The listing builds one solid part. Answer for the finished solid, in the listing's coordinates (mm). A direction names the side the tool comes from. Round coordinates to 2 decimals unless told otherwise and drop trailing zeros. Write each loop counter-clockwise with the first axis right and the second up, starting at its lowest first coordinate (ties: lowest second). Pieces come first, ordered by that corner, then holes. Notation, with made-up numbers: (-1.75, -21.75) - (4.25, -21.75) arc R22 ccw to (4.25, 9.25) - close; hole circle Ø11 at (76.25, -21). An arc over 180 degrees is marked (long way). Answer as CSV lines item,"result". Start each with the question number.
Item 1: A cutting plane is placed at A-A on y = 20. Determine the outline of the cut face in (x, z), and give its area (3 significant figures).
Item 2: For a pull along Y with two mould halves and no side action, classify faces 1 (the flat face through (37.5, -1, 33)), 2 (the cylindrical face through (70.5, 71, 1.5)), 3 (the flat face through (-34.5, 0, 32)), 4 (the flat face through (-1, 37.5, 33)) as pulls with the +Y half, pulls with the -Y half, needs draft (parallel to the pull), parting line crosses it, or undercut.
Item 3: Straight lines are drawn through the part: line 1 along Y through (x, z) = (72, 1); line 2 along Y through (x, z) = (72.5, 2). For each, find the intervals that lie inside material, in ascending order. Write a range as [from, to].
Item 4: A cutting plane is placed at B-B on x = -72.5. Determine the outline of the cut face in (y, z), and give its area (3 significant figures).
Item 5: A cutting plane is placed at C-C on z = 21. Determine the outline of the cut face in (x, y).
Item 6: Flat-ended cylindrical pins translate along their axes: pin 1 (4 mm diameter, centred on y = -4, z = 16, fed in from -X); pin 2 (4 mm diameter, centred on x = -29.5, z = 31.5, fed in from +Y); pin 3 (18 mm diameter, centred on x = -18.5, z = 42.5, fed in from -Y); pin 4 (6 mm diameter, centred on x = -72.5, y = -72.5, fed in from -Z). Find the tip coordinate at first contact, or state that the pin passes through.
Item 7: Which of the six approach directions +Z, -Z, +X, -X, +Y, -Y give full straight-line access (tool end or side, diameter ignored) to faces 5 (the flat face through (34.5, 0, 32)), 6 (the flat face through (-3, -36, 63)), 7 (the flat face through (-37.5, -1, 33)), 8 (the flat face through (-1, -37.5, 33))?
```python
from build123d import *

# Parameters (mm, degrees)
SKETCH_W     = 175
SKETCH_H     = 175
PAD_DEPTH    = 3
SKETCH001_R  = 2.5
HOLE_DEPTH   = 3.001
SKETCH002_W  = 75
SKETCH002_H  = 75
PAD001_DEPTH = 60
SKETCH003_W  = 69
SKETCH003_H  = 69
POCKET_DEPTH = 63.001


with BuildPart() as part:
    # Sketch → Pad (new body)
    with BuildSketch(Plane.XY):
        Rectangle(SKETCH_W, SKETCH_H)
    extrude(amount=PAD_DEPTH)

    # Sketch001 (on Face6 of Pad) → Hole (cut, through all)
    with BuildSketch(Plane.XY.offset(3)):
        with Locations((-72.5, 72.5)):
            Circle(SKETCH001_R)
        with Locations((72.5, 72.5)):
            Circle(SKETCH001_R)
        with Locations((-72.5, -72.5)):
            Circle(SKETCH001_R)
        with Locations((72.5, -72.5)):
            Circle(SKETCH001_R)
    extrude(amount=-HOLE_DEPTH, mode=Mode.SUBTRACT)

    # Sketch002 (on Face5 of Hole) → Pad001 (join)
    with BuildSketch(Plane.XY.offset(3)):
        Rectangle(SKETCH002_W, SKETCH002_H)
    extrude(amount=PAD001_DEPTH)

    # Sketch003 (on Face15 of Pad001) → Pocket (cut, through all)
    with BuildSketch(Plane.XY.offset(63)):
        Rectangle(SKETCH003_W, SKETCH003_H)
    extrude(amount=-POCKET_DEPTH, mode=Mode.SUBTRACT)


solid = part.part
```
Geometry says:
1,outline,"(-87.5, 0) - (-34.5, 0) - (-34.5, 63) - (-37.5, 63) - (-37.5, 3) - (-87.5, 3) - close; (34.5, 0) - (87.5, 0) - (87.5, 3) - (37.5, 3) - (37.5, 63) - (34.5, 63) - close"
1,area,"678 mm^2"
2,face 1,"needs draft"
2,face 2,"undercut"
2,face 3,"undercut"
2,face 4,"pulls with the +Y half"
3,line 1,"y = [-87.5, -74.95], [-70.05, 70.05], [74.95, 87.5]"
3,line 2,"y = [-87.5, -75], [-70, 70], [75, 87.5]"
4,outline,"(-87.5, 0) - (-75, 0) - (-75, 3) - (-87.5, 3) - close; (-70, 0) - (70, 0) - (70, 3) - (-70, 3) - close; (75, 0) - (87.5, 0) - (87.5, 3) - (75, 3) - close"
4,area,"495 mm^2"
5,outline,"(-37.5, -37.5) - (37.5, -37.5) - (37.5, 37.5) - (-37.5, 37.5) - close; hole (-34.5, -34.5) - (34.5, -34.5) - (34.5, 34.5) - (-34.5, 34.5) - close"
6,pin 1,"stops at x = -37.5"
6,pin 2,"stops at y = 37.5"
6,pin 3,"stops at y = -37.5"
6,pin 4,"stops at z = 0"
7,face 5,"+Z, -Z"
7,face 6,"+Z, +X, -X, +Y, -Y"
7,face 7,"+Z, -X, +Y, -Y"
7,face 8,"+Z, +X, -X, -Y"
